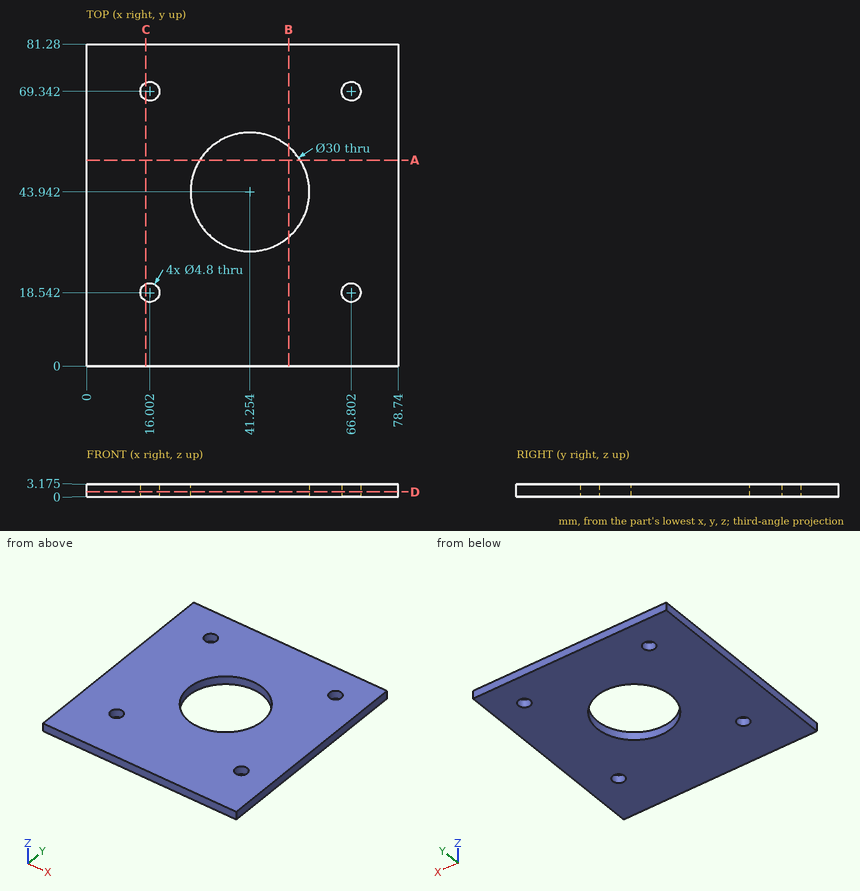
Input: dimensioned drawing with shaded views. Units: mm. Origin: part minimum x, y, z. Give positions to 0.01 mm unless a question says otherwise; leave off trailing zeros. Order: outer loops, then holes, each group sorted by start corner. A loop starts at its lowest first (then second) coordinate and runs counter-clockwise, first axis right, second up.
(1) Section query B-B (x = 51). Return the cut outline in (y, z) (3 decimals).
(2) Section query A-A (y = 52). Return the cut outline in (x, z) (3 decimals).
(3) Contact query for a flat-ended pin moving along its axis: P1, Ø4, axis at x = 50, y = 34.5, coming from the +Z side. Output: stop coordinate, or through.
(4) Material intervals for line 1 along X through (y, z) = (16.5, 1.25); line 2 along Y through (x, z) = (41.5, 1.4); line 3 along X through (y, z) = (55, 2.9), sorted ascending.
(5) Section query D-D (z = 1.2). Return the cut outline in (x, y).
(6) Section query C-C (x = 15). Return the cut outline in (y, z) (3 decimals), plus the area to 3 significant figures.
Outcome:
1. outline: (0, 0) - (32.54, 0) - (32.54, 3.175) - (0, 3.175) - close; (55.344, 0) - (81.28, 0) - (81.28, 3.175) - (55.344, 3.175) - close
2. outline: (0, 0) - (28.602, 0) - (28.602, 3.175) - (0, 3.175) - close; (53.906, 0) - (78.74, 0) - (78.74, 3.175) - (53.906, 3.175) - close
3. P1: passes through
4. line 1: x = 0 to 14.74, 17.26 to 65.54, 68.06 to 78.74
4. line 2: y = 0 to 28.94, 58.94 to 81.28
4. line 3: x = 0 to 31.12, 51.39 to 78.74
5. outline: (0, 0) - (78.74, 0) - (78.74, 81.28) - (0, 81.28) - close; hole circle Ø4.8 at (16, 18.54); hole circle Ø4.8 at (16, 69.34); hole circle Ø30 at (41.25, 43.94); hole circle Ø4.8 at (66.8, 18.54); hole circle Ø4.8 at (66.8, 69.34)
6. outline: (0, 0) - (16.361, 0) - (16.361, 3.175) - (0, 3.175) - close; (20.723, 0) - (67.161, 0) - (67.161, 3.175) - (20.723, 3.175) - close; (71.523, 0) - (81.28, 0) - (81.28, 3.175) - (71.523, 3.175) - close
6. area: 230 mm2
